```python
from build123d import *

# Parameters (mm, degrees)
SKETCH1_R           = 15.5
BOSS_EXTRUDE1_DEPTH = 12
SKETCH2_R           = 2.75
CUT_EXTRUDE1_DEPTH  = 25.989997999
SKETCH3_R           = 4.25
CUT_EXTRUDE2_DEPTH  = 25.989997999
CUT_EXTRUDE3_DEPTH  = 7.4
SKETCH5_R           = 5
CUT_EXTRUDE4_DEPTH  = 4
CHAMFER1_SIZE       = 0.5


with BuildPart() as part:
    # Sketch1 → Boss-Extrude1 (new body)
    with BuildSketch(Plane(origin=(0, 0, 0), x_dir=(1, 0, 0), z_dir=(0, 1, 0))):
        with Locations(Location((0, 0, 0), (0, 0, 270))):
            Circle(SKETCH1_R)
    extrude(amount=BOSS_EXTRUDE1_DEPTH)

    # Sketch2 → Cut-Extrude1 (cut, through all)
    with BuildSketch(Plane(origin=(0, 12, 0), x_dir=(1, 0, 0), z_dir=(0, 1, 0))):
        with Locations(Location((0, 10, 0), (0, 0, 270))):
            Circle(SKETCH2_R)
        with Locations(Location((0, -10, 0), (0, 0, 270))):
            Circle(SKETCH2_R)
    extrude(amount=-CUT_EXTRUDE1_DEPTH, mode=Mode.SUBTRACT)

    # Sketch3 → Cut-Extrude2 (cut, through all)
    with BuildSketch(Plane(origin=(0, 12, 0), x_dir=(1, 0, 0), z_dir=(0, 1, 0))):
        with Locations(Location((0, 0, 0), (0, 0, 270))):
            Circle(SKETCH3_R)
    extrude(amount=-CUT_EXTRUDE2_DEPTH, mode=Mode.SUBTRACT)

    # Sketch4 → Cut-Extrude3 (cut)
    with BuildSketch(Plane.XZ):
        Polygon((3.798941201, -6.539983111), (7.563262114, 0.019988032), (3.764320914, 6.559971143), (-3.798941201, 6.539983111), (-7.563262114, -0.019988032), (-3.764320914, -6.559971143), align=None)
    extrude(amount=-CUT_EXTRUDE3_DEPTH, mode=Mode.SUBTRACT)

    # Sketch5 → Cut-Extrude4 (cut)
    with BuildSketch(Plane(origin=(0, 12, 0), x_dir=(1, 0, 0), z_dir=(0, 1, 0))):
        with Locations(Location((0, 10, 0), (0, 0, 270))):
            Circle(SKETCH5_R)
        with Locations(Location((0, -10, 0), (0, 0, 270))):
            Circle(SKETCH5_R)
    extrude(amount=-CUT_EXTRUDE4_DEPTH, mode=Mode.SUBTRACT)

    # Chamfer1
    # the kernel refuses this chamfer: 0.5 mm, written as the material it takes off along each edge
    with BuildSketch(Plane(origin=(0, 12, 0), x_dir=(0, 0, 1), z_dir=(-1, 0, 0))) as chamfer1_piece_1:
        Polygon((4.25 + CHAMFER1_SIZE, 0), (4.25, -CHAMFER1_SIZE), (4.25, 0), align=None)
    revolve(axis=Axis((0, 12, 0), (0, 1, 0)), mode=Mode.SUBTRACT)
    with BuildSketch(Plane(origin=(0, 12, 0), x_dir=(0, 0, 1), z_dir=(-1, 0, 0))) as chamfer1_piece_2:
        Polygon((15.5, -CHAMFER1_SIZE), (15.5 - CHAMFER1_SIZE, 0), (15.5, 0), align=None)
    revolve(axis=Axis((0, 12, 0), (0, 1, 0)), mode=Mode.SUBTRACT)
    with BuildSketch(Plane(origin=(0, 12, -10), x_dir=(0, 0, 1), z_dir=(-1, 0, 0))) as chamfer1_piece_3:
        Polygon((5 + CHAMFER1_SIZE, 0), (5, -CHAMFER1_SIZE), (5, 0), align=None)
    revolve(axis=Axis((0, 12, -10), (0, 1, 0)), mode=Mode.SUBTRACT)
    with BuildSketch(Plane(origin=(0, 12, 10), x_dir=(0, 0, 1), z_dir=(-1, 0, 0))) as chamfer1_piece_4:
        Polygon((5 + CHAMFER1_SIZE, 0), (5, -CHAMFER1_SIZE), (5, 0), align=None)
    revolve(axis=Axis((0, 12, 10), (0, 1, 0)), mode=Mode.SUBTRACT)


solid = part.part
```
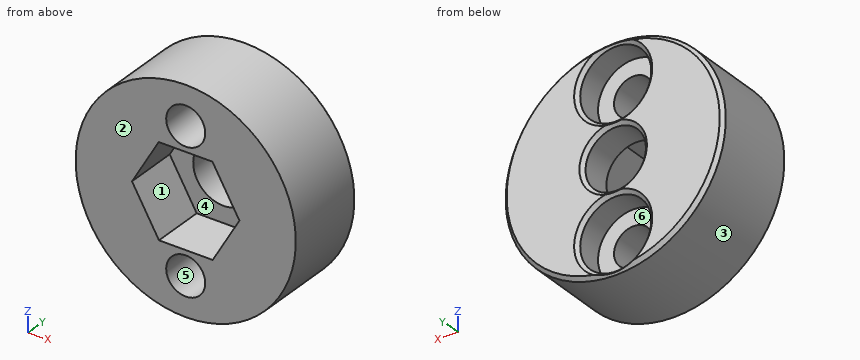
Check sheet for the modelled part. Datum: model origin and axes. Units: mm. Face numbers are marked on the shaded views. A direction names the side the tool comes from. Round coordinates to 2 decimals unless told otherwise and drop trailing zeros. Loops run counter-clockwise (first coordinate to the right, second up) from the corner with the lowest first, then second, coordinate; pieces in that order, holes last. Notation, with made-up numbers: (54.5, -17.75) -> (58.5, -17.75) arc R3 cw to (58.5, -12.75) -> close; hole circle Ø7 at (-13, -29). An arc over 180 degrees is marked (long way). Answer in a Markdown table with one row per item.
Q1. Set-up check for the marked faces 4, 5 and 6: record each of +Z, -Z, +X, -X, +Y, -Y from which the full face is reachable in a straight line by a thin tool's end or side.
Data:
| item | result |
|---|---|
| face 4 | -Y |
| face 5 | +Y, -Y |
| face 6 | +Y |
Q2. Sectioned sample at B-B on x = 0. Give the number of separate pieces and of enclosed holes in the cut face, then the cut area to 3 significant figures.
Data:
| item | result |
|---|---|
| separate pieces | 4 |
| enclosed holes | 0 |
| area | 67.1 mm^2 |
Q3. Thickness scan on L1, parallel to Z at x = 2, y = 5.25; L2, parallel to Z at x = -2.5, y = 1; L3, parallel to X at y = 9.6, z = 0. Record the ranges inside material, lowest first.
Data:
| item | result |
|---|---|
| L1 | z = -15.37 to -11.89, -8.11 to -6.54, 6.56 to 8.11, 11.89 to 15.37 |
| L2 | z = -15.3 to -11.15, -8.85 to -6.56, 6.54 to 8.85, 11.15 to 15.3 |
| L3 | x = -15.5 to -4.25, 4.25 to 15.5 |
Q4. Release check for a two-part mould opening along X. For the marked faces 1, 2 and 3 record: released by +X, released by -X, zero draft, split by the parting line, or undercut.
Data:
| item | result |
|---|---|
| face 1 | undercut |
| face 2 | zero draft |
| face 3 | split by the parting line |
Q5. Sectioned sample at A-A on y = 4.5. Enter the section's corners in (x, z).
Data:
| item | result |
|---|---|
| outline | circle Ø31 at (0, 0); hole (-7.56, -0.02) -> (-3.76, -6.56) -> (3.8, -6.54) -> (7.56, 0.02) -> (3.76, 6.56) -> (-3.8, 6.54) -> close; hole circle Ø5.5 at (0, -10); hole circle Ø5.5 at (0, 10) |
Q6. Go/stop test with flat-tipped pins: P1, Ø6, axis at x = 0, z = 10, coming from the +Y side; P2, Ø11.5, axis at x = 0, z = -10, coming from the -Y side; P3, Ø4, axis at x = -2.5, z = -2.5, coming from the -Y side; P4, Ø5, axis at x = -2.5, z = -10.5, coming from the +Y side. Record where each tip stops, or that it passes through.
Data:
| item | result |
|---|---|
| P1 | stops at y = 8 |
| P2 | stops at y = 0 |
| P3 | stops at y = 7.4 |
| P4 | stops at y = 11.55 |
